The listing builds one solid part. Answer for the finished solid, in the listing's coordinates (mm). Give positions to 0.01 mm unless a question says otherwise; leave off trailing zeros. Loops run counter-clockwise (first coordinate to the right, second up) from the corner with the lowest first, then second, coordinate; pieces in that order, holes last. Notation, with made-up numbers: (82.5, 45.25) - (112.5, 45.25) arc R19 cw to (112.5, 55.25) - close; hole circle Ø11 at (43, 4). An arc over 180 degrees is marked (long way). Write each question's results on one line, items separated by ' | '.
from build123d import *

# Parameters (mm, degrees)
F0_R     = 19.744958
F1_DEPTH = 19.005943
F2_R     = 5.08
F3_SIZE  = 5.08


with BuildPart() as f1:
    # F0 (on Front) → F1 (new body, symmetric)
    with BuildSketch(Plane.XZ):
        Polygon((41.21972, -43.068756), (57.908497, 14.162947), (16.688777, 57.231702), (-41.21972, 43.068756), (-57.908497, -14.162947), (-16.688777, -57.231702), align=None)
        Circle(F0_R, mode=Mode.SUBTRACT)
    extrude(amount=F1_DEPTH, both=True)

    # F2
    f2_edges = [f1.edges().sort_by_distance(p)[0] for p in [
        (-19.744958, -19.005943, 0),
    ]]
    fillet(f2_edges, radius=F2_R)

    # F3
    f3_edges = [f1.edges().sort_by_distance(p)[0] for p in [
        (-19.744958, 19.005943, 0),
    ]]
    chamfer(f3_edges, length=F3_SIZE)


solid = f1.part
Item 1: Find the intervals of material crossed by line 1 along X through (y, z) = (15.5, 12); line 2 along Z through (x, y) = (0, -3.5); line 3 along X through (y, z) = (-17, -3.5), in increasing order. Write a range as [from, to].
Values found:
line 1: x = [-50.28, -17.62], [17.62, 57.28] | line 2: z = [-53.15, -19.74], [19.74, 53.15] | line 3: x = [-54.8, -20.48], [20.48, 52.76]
Item 2: A cutting plane is placed at D-D, the plane z = 47. Determine the outline of the cut face in (x, y).
Values found:
outline: (-25.15, -19.01) - (26.48, -19.01) - (26.48, 19.01) - (-25.15, 19.01) - close
Item 3: Flat-ended cylindrical pins translate along their axes: P1, Ø5, axis at y = -3, z = 16.5, coming from the -X side; P2, Ø10, axis at x = -6, y = 8.5, coming from the +Z side; P3, Ø1, axis at x = -19, y = -14, coming from the +Z side; P4, Ø12, axis at x = -40.5, z = -39, coming from the -Y side. Find the tip coordinate at first contact, or state that the pin passes through.
Values found:
P1: stops at x = -49.7 | P2: stops at z = 52.91 | P3: stops at z = 48.63 | P4: stops at y = -19.01
Item 4: A cutting plane is placed at C-C, the plane x = 0. Determine the outline of the cut face in (y, z).
Values found:
outline: (-19.01, -53.15) - (19.01, -53.15) - (19.01, -24.82) - (13.93, -19.74) - (-13.93, -19.74) arc R5.08 ccw to (-19.01, -24.82) - close; (-19.01, 24.82) arc R5.08 ccw to (-13.93, 19.74) - (13.93, 19.74) - (19.01, 24.82) - (19.01, 53.15) - (-19.01, 53.15) - close
Item 5: A cutting plane is placed at A-A, the plane y = -0.5. Determine the outline of the cut face in (x, z), plus the area to 3 significant figures.
Values found:
outline: (-57.91, -14.16) - (-16.69, -57.23) - (41.22, -43.07) - (57.91, 14.16) - (16.69, 57.23) - (-41.22, 43.07) - close; hole circle Ø39.49 at (0, 0) | area: 8,010 mm²
Item 6: For a pull along X with two mould halves and no side action, classify faces 1 (the face through (37.587, -0.266, 35.396)), 2 (the face through (18.833, 0.195, 5.931)), 3 (the face through (-11.86, -0.27, 50.25)) as released by +X, released by -X, zero draft, split by the parting line, or undercut.
Values found:
face 1: released by +X | face 2: undercut | face 3: released by -X
Item 7: A cutting plane is placed at B-B, the plane z = 0. Determine the outline of the cut face in (x, y).
Values found:
outline: (-53.78, -19.01) - (-24.82, -19.01) arc R5.08 ccw to (-19.74, -13.93) - (-19.74, 13.93) - (-24.82, 19.01) - (-53.78, 19.01) - close; (19.74, -13.93) arc R5.08 ccw to (24.82, -19.01) - (53.78, -19.01) - (53.78, 19.01) - (24.82, 19.01) - (19.74, 13.93) - close
